For this review, take the finished solid that the model builds, in its own axes (mm). Face numbers are marked on the shaded views. Give positions to 0.01 mm unless a question says otherwise; leave off trailing zeros. Order: outer loops, then holes, each group sorted by start corner. A loop starts at its lowest first (then second) coordinate and runs counter-clockwise, first axis right, second up. Notation, with made-up numbers: (46.25, 72) - (97.25, 72) arc R22 ccw to (97.25, 99) - close; hole circle Ø4 at (60, 54.25). An arc over 180 degrees is marked (long way). Put each result on its own line as item: value. Start each with the question number.
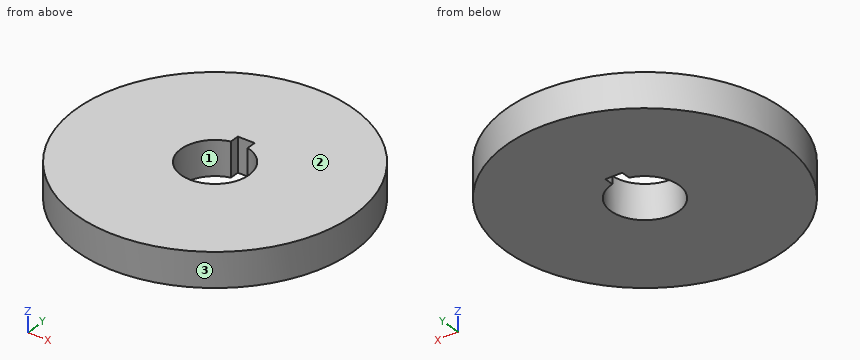
```python
from build123d import *

# Parameters (mm, degrees)
SKETCH1_R           = 25.75
BOSS_EXTRUDE1_DEPTH = 6.35


with BuildPart() as part:
    # Sketch1 → Boss-Extrude1 (new body)
    with BuildSketch(Plane.XY):
        Circle(SKETCH1_R)
        with BuildLine():
            Line((-1.5625, 7.875), (1.5625, 7.875))
            Line((1.5625, 7.875), (1.5625, 6.116064911))
            ThreePointArc((1.5625, 6.116064911), (0, -6.3125), (-1.5625, 6.116064911))
            Line((-1.5625, 6.116064911), (-1.5625, 7.875))
        make_face(mode=Mode.SUBTRACT)
    extrude(amount=BOSS_EXTRUDE1_DEPTH)


solid = part.part
```
1. Wall thickness on line 1 (X direction, y = -5.5, z = 1); line 2 (Y direction, x = 4, z = 4.75); line 3 (X direction, y = -2.5, z = 3.5): over which ranges is each line inside the solid? List them lowest first. Write a range as from..to.
2. Clearance check with flat-ended pins moving along their axes: pin 1 (3.5 mm diameter, centred on x = 0, z = 5, fed in from -Y); pin 2 (1.9 mm diameter, centred on y = 7, z = 4.5, fed in from -X); pin 3 (1.5 mm diameter, centred on x = -20.5, z = 3.5, fed in from -Y); pin 4 (10 mm diameter, centred on x = 0, y = 0, fed in from +Z). State where each tip first meets the part, or that it passes through.
3. The part is to be moulded in two halves that separate along X. For the marked faces 1, 2 and 3, say which applies: released by +X, released by -X, zero draft, split by the parting line, or undercut.
4. Add section B-B, the plane y = 0. Give the boundary of the cut face in (x, z), then the cut area to 3 significant figures.
5. Add section D-D, the plane x = -21.5. Give the boundary of the cut face in (y, z), then the cut area to 3 significant figures.
Found:
1. line 1: x = -25.16..-3.1, 3.1..25.16
1. line 2: y = -25.44..-4.88, 4.88..25.44
1. line 3: x = -25.63..-5.8, 5.8..25.63
2. pin 1: stops at y = -25.75
2. pin 2: stops at x = -25.03
2. pin 3: stops at y = -16.52
2. pin 4: passes through
3. face 1: undercut
3. face 2: zero draft
3. face 3: split by the parting line
4. outline: (-25.75, 0) - (-6.31, 0) - (-6.31, 6.35) - (-25.75, 6.35) - close; (6.31, 0) - (25.75, 0) - (25.75, 6.35) - (6.31, 6.35) - close
4. area: 247 mm^2
5. outline: (-14.17, 0) - (14.17, 0) - (14.17, 6.35) - (-14.17, 6.35) - close
5. area: 180 mm^2
